```python
from build123d import *

# Parameters (mm, degrees)
F1_DEPTH  = 6
F3_DEPTH  = 1
F7_W      = 42.1100177336
F7_H      = 2.7686282992
F7_W_2    = 43.2923636399
F7_H_2    = 2.6041977108
F8_DEPTH  = 25
F10_DEPTH = 3
F12_DEPTH = 3


with BuildPart() as f1:
    # F0 (on Top) → F1 (new body)
    with BuildSketch(Plane.XY):
        with BuildLine():
            Line((0, 7), (0, 0))
            Line((0, 0), (9, 0))
            ThreePointArc((9, 0), (9.7071067812, 0.2928932188), (10, 1))
            Line((10, 1), (10, 2.5))
            Line((10, 2.5), (8.6160635799, 2.5))
            Line((8.6160635799, 2.5), (8.6160635799, 1.5))
            Line((8.6160635799, 1.5), (7.6160635799, 1.5))
            Line((7.6160635799, 1.5), (7.6160635799, 2.5))
            Line((7.6160635799, 2.5), (3, 2.5))
            Line((3, 2.5), (3, 17.5))
            Line((3, 17.5), (7.6160635799, 17.5))
            Line((7.6160635799, 17.5), (7.6160635799, 18.5))
            Line((7.6160635799, 18.5), (8.6160635799, 18.5))
            Line((8.6160635799, 18.5), (8.6160635799, 17.5))
            Line((8.6160635799, 17.5), (10, 17.5))
            Line((10, 17.5), (10, 19))
            ThreePointArc((10, 19), (9.7071067812, 19.7071067812), (9, 20))
            Line((9, 20), (0, 20))
            Line((0, 20), (0, 13))
            Line((0, 13), (0, 7))
        make_face()
    extrude(amount=F1_DEPTH)

    # F2 (on face) → F3 (join)
    with BuildSketch(Plane(origin=(0, 0, 0), x_dir=(1, 0, 0), z_dir=(0, 0, -1))):
        with BuildLine():
            Line((10, -19), (10, -1))
            ThreePointArc((10, -1), (9.7071067812, -0.2928932188), (9, 0))
            Line((9, 0), (0, 0))
            Line((0, 0), (0, -20))
            Line((0, -20), (9, -20))
            ThreePointArc((9, -20), (9.7071067812, -19.7071067812), (10, -19))
        make_face()
    extrude(amount=-F3_DEPTH)

    # F5 (on offset) → F6 (revolve)
    with BuildSketch(Plane(origin=(0, 0, 3), x_dir=(1, 0, 0), z_dir=(0, 0, -1))):
        Polygon((-5.5, -7), (-5.5, -10), (0, -10), (0, -7), (-1.5, -7), (-1.5, -4.5), (-3, -4.5), align=None)
    revolve(axis=Axis((-2.75, 10, 3), (-1, 0, 0)))

    # F7 (on face) → F8 (cut)
    with BuildSketch(Plane(origin=(-5.5, 0, 0), x_dir=(0, -1, 0), z_dir=(-1, 0, 0))):
        with Locations((-5.2348260069, -1.3843141496)):
            Rectangle(F7_W, F7_H)
        with Locations((-5.5655788165, 7.3020988554)):
            Rectangle(F7_W_2, F7_H_2)
    extrude(amount=-F8_DEPTH, mode=Mode.SUBTRACT)

    # F9 (on face) → F10 (join)
    with BuildSketch(Plane(origin=(0, 0, 0), x_dir=(1, 0, 0), z_dir=(0, 0, -1))):
        Polygon((-5.5, -7), (-5.5, -10), (0, -10), (0, -7), (-1.5, -7), (-1.5, -4.5), (-3, -4.5), align=None)
    extrude(amount=-F10_DEPTH)

    # F11 (on face) → F12 (join)
    with BuildSketch(Plane.XY.offset(6)):
        Polygon((-5.5, 13), (-5.5, 10), (0, 10), (0, 13), (-1.5, 13), (-1.5, 15.5), (-3, 15.5), align=None)
    extrude(amount=-F12_DEPTH)


solid = f1.part
```
Read the model definition and answer for the solid it produces. Units are mm, in the model's axes. A direction names the side the tool comes from. Give positions to 0.01 mm unless a question says otherwise; leave off trailing zeros. Write each loop counter-clockwise with the first axis right and the second up, starting at its lowest first coordinate (ties: lowest second). Pieces come first, ordered by that corner, then holes. Notation, with made-up numbers: M 20.5,50.5 L 74.5,50.5 A16 ccw 74.5,74.5 Z; hole C -1.5,29.5 d7. An arc over 180 degrees is marked long. Put each result on its own line as item: value. Start each with the question number.
1. The part is cut by section A-A, the plane x = 5.5. Give the vertices of the cut face in (y, z).
2. For a pull along X with two mould halves and no side action, classify faces 5 (the flat face through (8.616, 2, 3)), 6 (the flat face through (3, 10, 3)), 7 (the flat face through (-2, 15.5, 5)) as released by +X, released by -X, zero draft, split by the parting line, or undercut.
3. The part is cut by section C-C, the plane x = 8. Give the vertices of the cut face in (y, z).
4. Which of the six approach directions +Z, -Z, +X, -X, +Y, -Y give full straight-line access (tool end or side, diameter ignored) to faces 1 (the flat face through (5, 17.5, 3)), 2 (the cylindrical face through (-0.76, 12.14, 0.9)), 3 (the cylindrical face through (-0.76, 7.86, 5.1)), 4 (the flat face through (8, 1.5, 3))?
5. Each of these flat-tipped pins is pushed along its axis until it touches: pin 1 Ø0.8 at (y, z) = (18, 3) entering from -X; pin 2 Ø0.8 at (x, z) = (-0.5, 1.5) entering from -Y; pin 3 Ø2 at (y, z) = (5.5, 2.5) entering from +X; pin 4 Ø3 at (y, z) = (13.5, 1.5) entering from +X. Where does it stop, or does it pass through?
6. Consider line 1 along Y through (x, z) = (6.25, 5.8); line 2 along Y through (x, z) = (8.25, 1.35); line 3 along X through (y, z) = (12, 3.65). Determine where each line is inside the solid, lowest interval first.
7. The part is cut by section B-B, the plane y = 4. Give the vertices of the cut face in (x, z).
Final values:
1. outline: M 0,0 L 20,0 L 20,6 L 17.5,6 L 17.5,1 L 2.5,1 L 2.5,6 L 0,6 Z
2. face 5: undercut
2. face 6: released by +X
2. face 7: zero draft
3. outline: M 0,0 L 20,0 L 20,6 L 18.5,6 L 18.5,1 L 1.5,1 L 1.5,6 L 0,6 Z
4. face 1: +Z, +X
4. face 2: -Z, +Y
4. face 3: +Z, -Y
4. face 4: +Z
5. pin 1: stops at x = 0
5. pin 2: stops at y = 7
5. pin 3: stops at x = 3
5. pin 4: stops at x = 10
6. line 1: y = 0 to 2.5, 17.5 to 20
6. line 2: y = 0 to 1.5, 18.5 to 20
6. line 3: x = -5.5 to 3
7. outline: M 0,0 L 10,0 L 10,1 L 3,1 L 3,6 L 0,6 Z
